Check sheet for the modelled part. Datum: model origin and axes. Units: mm. Face numbers are marked on the shaded views. A direction names the side the tool comes from. Round coordinates to 2 decimals unless told otherwise and drop trailing zeros. Loops run counter-clockwise (first coordinate to the right, second up) from the corner with the lowest first, then second, coordinate; pieces in that order, holes last. Notation, with made-up numbers: (48, -35.75) - (56, -35.75) arc R20 cw to (56, 0.25) - close; hole circle Ø8 at (-20.5, 0.5). An arc over 180 degrees is marked (long way). Answer in a Markdown table with one row per item. Add a question column.
(1) Cross-section at B-B on x = -16. Enter the section's corners in (y, z), then the cut area to 3 significant figures.
(2) Cross-section at A-A on x = -65. Enter the section's corners in (y, z).
(3) Gauge pin test, flat ends, axial feed: pin 1 (10 mm diameter, centred on x = 23.5, z = 1, fed in from -Y); pin 2 (4 mm diameter, centred on y = 77.5, z = 0.5, fed in from -X); pin 3 (5 mm diameter, centred on x = 20, z = 71.5, fed in from +Y); pin 4 (5 mm diameter, centred on y = 17.5, z = -38, fed in from +X). Record the tip position at first contact, or that the pin passes through.
(4) Thickness scan on line 1 along Y through (x, z) = (-65, 0); line 2 along Y through (x, z) = (31, 0); line 3 along Z through (x, y) = (8, -19). Record the ranges inside material, lowest first.
(5) Access from +Z, -Z, +X, -X, +Y, -Y to the whole of each face (thin tool, end or side, straight path). Record for the marked faces 1 and 2.
(6) Mould release check, pull along Y, two halves, no side actions. Record for the marked faces 3, 4 and 5: +Y half, -Y half, draft (parallel to the pull), parting line (faces both ways), or undercut.
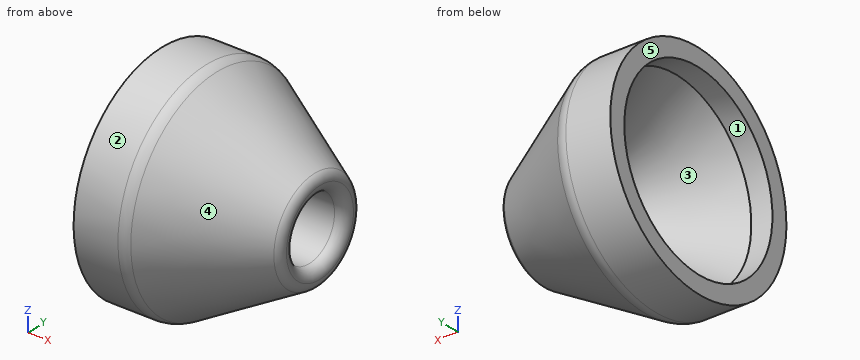
from build123d import *


with BuildPart() as f1:
    # F0 (on Front) → F1 (revolve)
    with BuildSketch(Plane.XZ):
        with BuildLine():
            Line((-32.942286, 105), (-75, 105))
            Line((-75, 105), (-75, 88.320389))
            Line((-75, 88.320389), (-55, 88.320389))
            Line((-55, 88.320389), (18.318778, 30))
            Line((18.318778, 30), (65, 30))
            ThreePointArc((65, 30), (72.071068, 32.928932), (75, 40))
            ThreePointArc((75, 40), (73.660254, 45), (70, 48.660254))
            Line((70, 48.660254), (-22.942286, 102.320508))
            ThreePointArc((-22.942286, 102.320508), (-27.765905, 104.318517), (-32.942286, 105))
        make_face()
    revolve(axis=Axis((-37.41489, 0, 0), (-1, 0, 0)))


solid = f1.part
Answers:
| question | item | result |
|---|---|---|
| 1 | outline | circle Ø196.62 at (0, 0); hole circle Ø114.6 at (0, 0) |
| 1 | area | 20,100 mm^2 |
| 2 | outline | circle Ø210 at (0, 0); hole circle Ø176.64 at (0, 0) |
| 3 | pin 1 | stops at y = -78.39 |
| 3 | pin 2 | stops at x = -43.91 |
| 3 | pin 3 | stops at y = 36.28 |
| 3 | pin 4 | stops at x = 75 |
| 4 | line 1 | y = -105 to -88.32, 88.32 to 105 |
| 4 | line 2 | y = -71.18 to -30, 30 to 71.18 |
| 4 | line 3 | z = -82.29 to -33.15, 33.15 to 82.29 |
| 5 | face 1 | -X |
| 5 | face 2 | +X, -X |
| 6 | face 3 | undercut |
| 6 | face 4 | parting line |
| 6 | face 5 | draft |
